Autodesk Inventor part; units mm, degrees
ref_plane "YZ Plane" through (0, 0, 0) normal (1, 0, 0) x (0, 1, 0)
ref_plane "XZ Plane" through (0, 0, 0) normal (0, 1, 0) x (-1, 0, 0)
ref_plane "XY Plane" through (0, 0, 0) normal (0, 0, 1) x (1, 0, 0)
ref_plane "Arbeitsebene1" through (0, 0, 0) normal (0, 0, 1) x (1, 0, 0)
ref_plane "Arbeitsebene2" through (-25.4, 26.0506, 0) normal (-1, 0, 0) x (0, 0, 1)
sketch "Skizze2" plane through (-25.4, 26.0506, 0) normal (-1, 0, 0) x (0, 0, 1)
  line L0 (0, 0) -> (0, 32.2)
  line L1 (0, 24.2) -> (-26, 24.2)
  line L2 (-26, 24.2) -> (-26, -30.8)
  line L3 (-26, -30.8) -> (0, -30.8)
  line L4 (0, -30.8) -> (0, 24.2)
  line L5 (5, 0) -> (0, 0)
  line L6 (0, 0) -> (0, -30.8)
  line L7 (0, -30.8) -> (5, -30.8)
  point P0 (0, -26.0506)
  dimension "d26" = 26
  dimension "d27" = 55
extrude "Extrusion2" add sketch "Skizze2" against normal blind 8
ref_plane "Arbeitsebene3" through (0, 0, 5) normal (0, 0, 1) x (1, 0, 0)
sketch "Skizze6" plane through (0, 0, 5) normal (0, 0, 1) x (1, 0, 0)
  point P0 (0, 0)
ref_plane "Arbeitsebene4" through (0, 0, 5) normal (0, 0, 1) x (1, 0, 0)
ref_plane "Arbeitsebene5" through (-15, 26.0506, 0) normal (-1, 0, 0) x (0, 0, 1)
sketch "Skizze8" plane through (-15, 26.0506, 0) normal (-1, 0, 0) x (0, 0, 1)
  line L0 (-14, 32.2) -> (-14, 0)
  line L1 (0, 0) -> (-14, 0)
  line L2 (0, 32.2) -> (0, 0)
  line L3 (0, 32.2) -> (-14, 32.2)
  line L4 (-8.5, 27.35) -> (0, 27.35)
  line L5 (-8.5, 24.85) -> (0, 24.85)
  line L6 (-8.5, 7.35) -> (0, 7.35)
  line L7 (-8.5, 4.85) -> (0, 4.85)
  circle A0 centre (-7, 26.15) radius 1.6
  circle A1 centre (-7, 6.15) radius 1.6
  point P0 (0, -26.0506)
  dimension "d44" = 3.2
  dimension "d45" = 3.2
  dimension "d46" = 1.2
  dimension "d47" = 1.2
extrude "Extrusion6" add sketch "Skizze8" along normal up to surface (10.4 mm away) contours L3 L2 L4 A0 L5 L6 A1 L7 L1 L0 | L2 L5 A0 L4 | L7 A1 L6 L2
sketch "Skizze9" plane through (-25.4, 26.0506, 0) normal (-1, 0, 0) x (0, 0, 1)
  circle A0 centre (-7, 6.15) radius 1.6
  circle A1 centre (-7, 26.15) radius 1.6
  point P0 (0, -26.0506)
hole "Bohrung2" at (-25.4, 32.2006, -7) at (-25.4, 52.2006, -7) direction (1, 0, 0) diameter 3.2 end through all counterbore diameter 6.5 counterbore depth 5
sketch "Skizze7" plane through (0, 0, 5) normal (0, 0, 1) x (1, 0, 0)
  line L0 (15, 26.0506) -> (15, 58.2506)
  line L1 (15, 58.2506) -> (-25.4, 58.2506)
  line L2 (-25.4, 58.2506) -> (-25.4, -4.7494)
  line L3 (-25.4, -4.7494) -> (-17.4, -4.7494)
  line L4 (-17.4, 26.0506) -> (-17.4, -4.7494)
  line L5 (-17.4, 26.0506) -> (15, 26.0506)
  circle A0 centre (-21.4, 10.1506) radius 1.5
  circle A1 centre (-21.4, 26.1506) radius 1.4
  circle A2 centre (-21.4, 42.1506) radius 1.4
  point P0 (0, 0)
  dimension "d38" = 3
  dimension "d57" = 2.8
  dimension "d58" = 2.8
  dimension "d59" = 16
  dimension "d60" = 16
  dimension "d61" = 8
  dimension "d62" = 4
  dimension "d63" = 4
  dimension "d64" = 4
  dimension "d65" = 16.1
hole "Bohrung1" at (-21.4, 42.1506, 5) at (-21.4, 26.1506, 5) at (-21.4, 10.1506, 5) direction (0, 0, -1) diameter 3.2 end through all counterbore diameter 6.5 counterbore depth 20
sketch "Skizze10" plane through (-15, 26.0506, 0) normal (1, 0, 0) x (0, 0, -1)
  line L0 (0, 32.2) -> (14, 32.2)
  line L1 (14, 0) -> (14, 32.2)
  line L2 (0, 0) -> (0, 32.2)
  circle A0 centre (-2.5, 50.2) radius 1.5 construction
  circle A1 centre (12.5, 50.2) radius 1.5 construction
  line L3 (13, 67.2) -> (-3, 67.2)
  line L4 (-5, 66.0453) -> (-5, 48.3547)
  line L5 (14.75, 176.5265) -> (14.75, -9.4735)
  line L6 (-5, 32.2) -> (14.75, 32.2)
  line L7 (14.75, 32.2) -> (14.75, 67.2)
  line L8 (14.75, 67.2) -> (-5, 67.2)
  line L9 (-5, 67.2) -> (-5, 32.2)
  line L10 (10, 52.2) -> (10, 45.2)
  line L11 (10, 52.2) -> (8.35, 52.2)
  line L12 (0, 45.2) -> (0, 52.2)
  line L13 (10, 44.2036) -> (0, 44.2036)
  line L14 (0, 44.2036) -> (0, 57.2)
  line L15 (0, 57.2) -> (10, 57.2)
  line L16 (10, 57.2) -> (10, 44.2036)
  circle A2 centre (12.5, 50.2) radius 1.4
  circle A3 centre (-2.5, 50.2) radius 1.4
  line L17 (-5, 32.2) -> (0, 27.2)
  line L18 (0, -30.8) -> (0, 32.2)
  line L19 (-5, 32.2) -> (2.0711, 32.2) construction
  line L20 (0, 27.2) -> (0, 32.2)
  line L21 (14.75, 32.2) -> (14.75, 24.2)
  line L22 (26, 24.2) -> (14, 24.2)
  point P0 (0, -26.0506)
  point P1 (10, 45.2)
  point P2 (0, 32.2)
  point P3 (14.75, 32.2)
  point P4 (13, 67.2)
  point P5 (0, 27.2)
  dimension "d66" = 2.8
  dimension "d67" = 2.8
  dimension "d70" = 45
extrude "Extrusion7" [suppressed]
chamfer "Fase2" distance 5 angle 45 1 edges at (-21.4, -4.7494, 0)
properties part number "30_XYTable_Aliexpress_Translatorarm_x"
Check sheet for the modelled part. Datum: model origin and axes. Units: mm. A direction names the side the tool comes from. Round coordinates to 2 decimals unless told otherwise and drop trailing zeros. Loops run counter-clockwise (first coordinate to the right, second up) from the corner with the lowest first, then second, coordinate; pieces in that order, holes last. Notation, with made-up numbers: M -33.75,80.5 L 22.25,80.5 A14 ccw 22.25,89.5 Z; hole C 17.25,78 d7. An arc over 180 degrees is marked long. One line per item, written item: value.
(1) Depth check by flat-ended pin: pin 1 Ø13 at (y, z) = (14, -16.5) entering from +X; pin 2 Ø0.7 at (x, z) = (-16, -4.5) entering from -Y; pin 3 Ø3 at (x, y) = (-22.5, 26) entering from +Z. Enter the tip coordinate at first touch or a pass-through.
Computed values:
pin 1: stops at x = -17.4
pin 2: stops at y = 26.05
pin 3: stops at z = -15
(2) Thickness scan on line 1 (Y direction, x = -22.75, z = -11.75); line 2 (Y direction, x = -21.4, z = -6.75); line 3 (Y direction, x = -21.4, z = -22). Record the ranges inside material, lowest first.
Computed values:
line 1: y = -4.75 to 7.19, 13.11 to 23.19, 29.11 to 39.19, 45.11 to 58.25
line 2: y = -4.75 to 6.9, 13.4 to 22.9, 35.44 to 38.9, 45.4 to 48.96, 55.44 to 58.25
line 3: y = -4.75 to 8.55, 11.75 to 24.55, 27.75 to 40.55, 43.75 to 50.25
(3) Sectioned sample at B-B, the plane x = -21.4. Count the separate pieces of the cut face and the enclosed holes in it, then the cut area to 3 significant figures.
Computed values:
separate pieces: 4
enclosed holes: 1
area: 1,070 mm^2
(4) Sectioned sample at D-D, the plane y = 6. Record the cut outline in (x, z).
Computed values:
outline: M -25.4,-26 L -17.4,-26 L -17.4,0 L -25.4,0 Z
(5) Release check for a two-part mould opening along Z. For faces 1 (the face through (-21, 50.251, -20)), 2 (the face through (-19, 29, 0)), 3 (the face through (-22.865, 35.084, -5.5)) record: +Z half, -Z half, draft (parallel to the pull), parting line (faces both ways), or undercut.
Computed values:
face 1: draft
face 2: +Z half
face 3: undercut
(6) Access from +Z, -Z, +X, -X, +Y, -Y to the whole of each face (thin tool, end or side, straight path). Record for faces 4 (the face through (-18.23, 10.86, -7.6)), 5 (the face through (-20.4, 54, -6)), 6 (the face through (-17, 50, -14)), 7 (the face through (-16, 26.051, -7)), 8 (the face through (-20.4, 43.4, -20.6)).
Computed values:
face 4: +Z
face 5: -X
face 6: -Z, +X, +Y
face 7: +Z, -Z, +X, -Y
face 8: +Z, -Z
(7) Sectioned sample at A-A, the plane z = -7. Record the cut outline in (x, y), then the cut area to 3 significant figures.
Computed values:
outline: M -25.4,-4.75 L -17.4,-4.75 L -17.4,26.05 L -15,26.05 L -15,30.6 L -20.4,30.6 L -20.4,29.24 A3.25 cw long -23.05,28.95 L -25.4,28.95 Z; M -25.4,35.45 L -20.4,35.45 L -20.4,33.8 L -15,33.8 L -15,50.6 L -20.4,50.6 L -20.4,48.95 L -25.4,48.95 Z; M -25.4,55.45 L -20.4,55.45 L -20.4,53.8 L -15,53.8 L -15,58.25 L -25.4,58.25 Z; hole C -21.4,10.15 d6.5; hole C -21.4,42.15 d6.5
area: 383 mm^2
(8) Sectioned sample at C-C, the plane z = -24.5. Record the cut outline in (x, y), then the cut area to 3 significant figures.
Computed values:
outline: M -25.4,-4.75 L -17.4,-4.75 L -17.4,50.25 L -25.4,50.25 Z; hole C -21.4,10.15 d3.2; hole C -21.4,26.15 d3.2; hole C -21.4,42.15 d3.2
area: 416 mm^2
